from build123d import *

# Parameters (mm, degrees)
SKETCH1_R               = 2.38125
BOSS_EXTRUDE1_DEPTH     = 9.525
CUT_EXTRUDE1_DEPTH      = 51.855779923
CUT_EXTRUDE1_DEPTH_BACK = 51.855779923
SKETCH2_R               = 2.1828125
FILLET1_R               = 4.7625
CHAMFER1_SIZE           = 0.396875


with BuildPart() as part:
    # Sketch1 → Boss-Extrude1 (new body)
    with BuildSketch(Plane.XY):
        with BuildLine():
            Line((0, 0), (0, 15.08125))
            Line((0, 15.08125), (20.240625, 15.08125))
            ThreePointArc((20.240625, 15.08125), (24.730753061, 13.221378061), (26.590625, 8.73125))
            Line((26.590625, 8.73125), (26.590625, 4.7625))
            ThreePointArc((26.590625, 4.7625), (27.055592985, 3.639967985), (28.178125, 3.175))
            Line((28.178125, 3.175), (47.625, 3.175))
            Line((47.625, 3.175), (47.625, 0))
            Line((47.625, 0), (0, 0))
        make_face()
        with Locations(Location((20.240625, 8.73125, 0), (0, 0, 180))):
            Circle(SKETCH1_R, mode=Mode.SUBTRACT)
    extrude(amount=BOSS_EXTRUDE1_DEPTH)

    # Sketch2 → Cut-Extrude1 (cut, two sides: drawn at the far end of the back side and taken through both)
    with BuildSketch(Plane(origin=(0, 15.08125, 0), x_dir=(1, 0, 0), z_dir=(0, 1, 0)).offset(-CUT_EXTRUDE1_DEPTH_BACK)):
        with Locations(Location((4.7625, -4.7625, 0), (0, 0, 270))):
            Circle(SKETCH2_R)
        with Locations(Location((42.8625, -4.7625, 0), (0, 0, 270))):
            Circle(SKETCH2_R)
    extrude(amount=CUT_EXTRUDE1_DEPTH + CUT_EXTRUDE1_DEPTH_BACK, mode=Mode.SUBTRACT)

    # Fillet1
    fillet1_edges = [part.edges().sort_by_distance(p)[0] for p in [
        (47.625, 1.5875, 9.525),
        (47.625, 1.5875, 0),
        (0, 7.540625, 0),
        (0, 7.540625, 9.525),
    ]]
    fillet(fillet1_edges, radius=FILLET1_R - 0.0001)  # a hair under: the kernel refuses the full size

    # Chamfer1
    chamfer1_edges = [part.edges().sort_by_distance(p)[0] for p in [
        (27.055592985, 3.639967985, 0),
        (27.055592985, 3.639967985, 9.525),
        (26.590625, 6.746875, 9.525),
        (22.621875, 8.73125, 0),
        (22.621875, 8.73125, 9.525),
        (24.730753061, 13.221378061, 9.525),
        (12.5015125, 15.08125, 9.525),
        (4.7625, 0, 2.5796875),
        (4.7625, 15.08125, 2.5796875),
        (42.8625, 0, 2.5796875),
        (42.8625, 3.175, 2.5796875),
        (23.8125, 0, 9.525),
        (35.5203625, 3.175, 9.525),
        (35.5203625, 3.175, 0),
        (46.230125335, 3.175, 1.394874665),
        (46.230125335, 3.175, 8.130125335),
        (23.8125, 0, 0),
        (1.394874665, 0, 8.130125335),
        (1.394874665, 0, 1.394874665),
        (46.230125335, 0, 1.394874665),
        (46.230125335, 0, 8.130125335),
        (1.394874665, 15.08125, 8.130125335),
        (1.394874665, 15.08125, 1.394874665),
        (12.5015125, 15.08125, 0),
        (24.730753061, 13.221378061, 0),
        (26.590625, 6.746875, 0),
    ]]
    chamfer(chamfer1_edges, length=CHAMFER1_SIZE)


solid = part.part
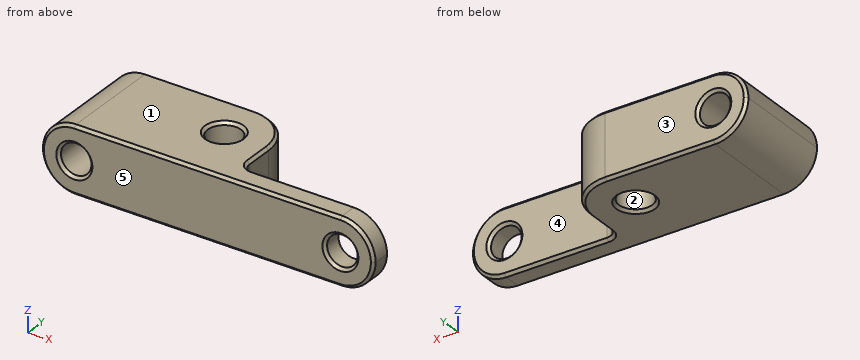
Source: CAD feature listing. Evaluate the final solid. Frame: model axes, mm. Face numbers are marked on the shaded views. A direction names the side the tool comes from. Give positions to 0.01 mm unless a question says otherwise; leave off trailing zeros. Loops run counter-clockwise (first coordinate to the right, second up) from the corner with the lowest first, then second, coordinate; pieces in that order, holes last. Notation, with made-up numbers: (-26, 61.25) -> (17, 61.25) arc R20 cw to (17, 98.25) -> close; hole circle Ø2 at (-37, 70). An arc over 180 degrees is marked (long way). Use a Markdown table: item, result. Add a question column.
1) Section query B-B, the plane z = 4. Count the separate pieces of the cut face and the enclosed holes in it, then the cut area to 3 significant figures.
2) First-contact query: pin 1 (4 mm diameter, centred on y = 7.5, z = 2, fed in from -X); pin 2 (2 mm diameter, centred on y = 6, z = 5, fed in from +X); pin 3 (1 mm diameter, centred on x = 40.5, z = 5, fed in from +Y) (3 decimals). Flat tips, straight axial feed; report the tip coordinate or a pass-through.
3) Line query: line 1 along X through (y, z) = (8.5, 5.5); line 2 along X through (y, z) = (8.75, 4.5); line 3 along X through (y, z) = (14, 4.25). Output: solid intervals per line, ascending. Write a range as [from, to].
4) Section query A-A, the plane x = 30.5. Return the cut outline in (y, z) (3 decimals).
5) Pull-direction query (Y, two-part tool) for the marked faces 1, 2 and 3; classes: +Y half, -Y half, draft (parallel to the pull), parting line (faces both ways), or undercut.
6) Reachability of the marked faces 4 and 5 from +Z, -Z, +X, -X, +Y, -Y: full face, straight path, thin tool, end or side. Return the list, or none.
Numbers:
| question | item | result |
|---|---|---|
| 1 | separate pieces | 3 |
| 1 | enclosed holes | 1 |
| 1 | area | 365 mm2 |
| 2 | pin 1 | stops at x = 0.06 |
| 2 | pin 2 | stops at x = 26.59 |
| 2 | pin 3 | stops at y = 3.175 |
| 3 | line 1 | x = [0.06, 2.71], [6.82, 17.87], [22.61, 26.59] |
| 3 | line 2 | x = [0.01, 2.6], [6.93, 17.86], [22.62, 26.59] |
| 3 | line 3 | x = [0.03, 2.64], [6.88, 23.79] |
| 4 | outline | (0, 0.397) -> (0.397, 0) -> (2.778, 0) -> (3.175, 0.397) -> (3.175, 9.128) -> (2.778, 9.525) -> (0.397, 9.525) -> (0, 9.128) -> close |
| 5 | face 1 | draft |
| 5 | face 2 | undercut |
| 5 | face 3 | +Y half |
| 6 | face 4 | +Z, -Z, +X, +Y |
| 6 | face 5 | +Z, -Z, +X, -X, -Y |
